from build123d import *

# Parameters (mm, degrees)
F0_W     = 12.7
F0_H     = 63.5
F1_DEPTH = 66.675
F0_W_2   = 101.6
F0_H_2   = 76.2
F0_R     = 3.9624
F2_DEPTH = 15.875
F3_R     = 3.048
F4_R     = 5.08
F6_W     = 6.35
F6_H     = 76.2
F7_DEPTH = 5.08
F5_R     = 12.7
F8_DEPTH = 37.592


with BuildPart() as f1:
    # F0 (on Top) → F1 (new body)
    with BuildSketch(Plane.XY):
        with Locations((-1.256721, 13.457914)):
            Rectangle(F0_W, F0_H)
    extrude(amount=F1_DEPTH)

    # F0 (on Top) → F2 (join)
    with BuildSketch(Plane.XY):
        with Locations((-1.256721, 12.390629)):
            Rectangle(F0_W_2, F0_H_2)
        with Locations((-39.873372, -14.794378)):
            Circle(F0_R, mode=Mode.SUBTRACT)
        with Locations((-40.350091, 39.065836)):
            Circle(F0_R, mode=Mode.SUBTRACT)
        with Locations((-1.256721, 13.457914)):
            Rectangle(F0_W, F0_H, mode=Mode.SUBTRACT)
    extrude(amount=F2_DEPTH)

    # F3
    f3_edges = [f1.edges().sort_by_distance(p)[0] for p in [
        (-1.256721, -18.292086, 66.675),
        (-1.256721, 45.207914, 66.675),
        (-1.256721, -18.292086, 15.875),
        (-1.256721, 45.207914, 15.875),
    ]]
    fillet(f3_edges, radius=F3_R)

    # F4
    f4_edges = [f1.edges().sort_by_distance(p)[0] for p in [
        (-52.056721, -25.709371, 7.9375),
        (49.543279, -25.709371, 7.9375),
        (49.543279, 50.490629, 7.9375),
        (-52.056721, 50.490629, 7.9375),
    ]]
    fillet(f4_edges, radius=F4_R)

    # F6 (on face) → F7 (cut)
    with BuildSketch(Plane(origin=(0, 0, 0), x_dir=(1, 0, 0), z_dir=(0, 0, -1))):
        with Locations((24.143279, -12.390629)):
            Rectangle(F6_W, F6_H)
    extrude(amount=-F7_DEPTH, mode=Mode.SUBTRACT)

    # F5 (on face) → F8 (cut)
    with BuildSketch(Plane.YZ.offset(5.093279)):
        with Locations((13.457914, 41.275)):
            Circle(F5_R)
    extrude(amount=-F8_DEPTH, mode=Mode.SUBTRACT)


solid = f1.part
Input: part model. Units: mm. Frame: model coordinates. A direction names the side the tool comes from. Coordinates: 2 decimals unless noted, no trailing zeros. Order: outer loops, then holes, each group sorted by start corner. A loop starts at its lowest first (then second) coordinate and runs counter-clockwise, first axis right, second up. Notation, with made-up numbers: M 71,10.5 L 94,10.5 A12 ccw 94,23.5 Z; hole C 19,10 d10. An arc over 180 degrees is marked long. Write item = value, one per line. Start each with the question number.
(1) Line query: line 1 along X through (y, z) = (27.5, 37.5); line 2 along Z through (x, y) = (14.5, 26) (3 decimals); line 3 along X through (y, z) = (8.5, 3). Output: solid intervals per line, ascending. Write a range as [from, to].
(2) Section C-C on x = -1. Output: boundary loops of the cut face in (y, z) (3 decimals).
(3) Pull-direction query (Y, two-part tool) for faces 1 (the cylindrical face through (-42.794, -12.116, 7.826)), 2 (the flat face through (-16, 13, 0)), 3 (the cylindrical face through (-50.53, -24.26, 8.05)); classes: released by +Y, released by -Y, zero draft, split by the parting line, or undercut.
(4) Reachability of faces 4 (the flat face through (49.543, 12, 8)), 5 (the flat face through (5.093, 5, 30)), 6 (the cylindrical face through (-1.2, 44.3, 65.8)), 7 (the flat face through (-7.607, 5, 30)), 8 (the flat face through (27.318, 13, 3)) from +Z, -Z, +X, -X, +Y, -Y: full face, straight path, thin tool, end or side. Return the list, or none.
(5) Section D-D on z = 10. Output: boundary loops of the cut face in (x, y).
(6) Section B-B on z = 38.5. Output: boundary loops of the cut face in (x, y), and give its area (3 significant figures).
(7) Section A-A on y = 24. Output: boundary loops of the cut face in (x, z) (3 decimals).
(8) First-contact query: P1, Ø4, axis at y = 23, z = 48.5, coming from the +X side; P2, Ø3, axis at x = 23, y = 23, coming from the -Z side; P3, Ø5, axis at x = 38.5, y = 12, coming from the +Z side (3 decimals); P4, Ø6.5, axis at x = -40.35, y = 39.07, coming from the +Z side. Flat tips, straight axial feed; report the tip coordinate or a pass-through.
Result set:
q1.line_1 = [-7.61, 5.09]
q1.line_2 = [0, 15.875]
q1.line_3 = [-52.06, 20.97], [27.32, 49.54]
q2.outline = M -25.709,0 L 50.491,0 L 50.491,15.875 L 48.256,15.875 A3.048 cw 45.208,18.923 L 45.208,63.627 A3.048 ccw 42.16,66.675 L -15.244,66.675 A3.048 ccw -18.292,63.627 L -18.292,18.923 A3.048 cw -21.34,15.875 L -25.709,15.875 Z; hole C 13.458,41.275 d25.4
q3.face_1 = undercut
q3.face_2 = zero draft
q3.face_3 = released by -Y
q4.face_4 = +Z, -Z, +X, +Y, -Y
q4.face_5 = +Z, +X, +Y, -Y
q4.face_6 = +Z, +X, -X, +Y
q4.face_7 = +Z, -X, +Y, -Y
q4.face_8 = -Z, +Y, -Y
q5.outline = M -52.06,-20.63 A5.08 ccw -46.98,-25.71 L 44.46,-25.71 A5.08 ccw 49.54,-20.63 L 49.54,45.41 A5.08 ccw 44.46,50.49 L -46.98,50.49 A5.08 ccw -52.06,45.41 Z; hole C -40.35,39.07 d7.92; hole C -39.87,-14.79 d7.92
q6.outline = M -7.61,-18.29 L 5.09,-18.29 L 5.09,1.06 L -7.61,1.06 Z; M -7.61,25.85 L 5.09,25.85 L 5.09,45.21 L -7.61,45.21 Z
q6.area = 492 mm²
q7.outline = M -52.057,0 L 20.968,0 L 20.968,5.08 L 27.318,5.08 L 27.318,0 L 49.543,0 L 49.543,15.875 L 5.093,15.875 L 5.093,34.193 L -7.607,34.193 L -7.607,15.875 L -52.057,15.875 Z; M -7.607,48.357 L 5.093,48.357 L 5.093,66.675 L -7.607,66.675 Z
q8.P1 = 5.09
q8.P2 = 5.08
q8.P3 = 15.875
q8.P4 = through
